Work out the finished part from the listing and answer in its coordinate system (mm). Face numbers are marked on the shaded views. A direction names the side the tool comes from. Coordinates: 2 decimals unless noted, no trailing zeros. Order: outer loops, then holes, each group sorted by start corner. A loop starts at its lowest first (then second) coordinate and runs counter-clockwise, first axis right, second up.
1. A tool of negligible diameter and unlimited length cuts with its end or side. For the marked faces 1 and 2, from which of +Z, -Z, +X, -X, +Y, -Y can it reach the whole face along a straight path? Write none if from no direction.
2. Find the intervals of material crossed by probe 1 along Y at (x, z) = (-5.5, 2); probe 2 along X at (y, z) = (0.5, 9); probe 3 along X at (y, z) = (4.25, 3.5), in increasing order.
3. The part is cut by section A-A, the plane y = 0. Give the vertices of the cut face in (x, z), then the cut area to 3 significant figures.
4. The part is cut by section B-B, the plane z = 3.5. Give the vertices of the cut face in (x, y), then the cut area to 3 significant figures.
5. Flat-ended cylindrical pins translate along their axes: pin 1 Ø4 at (y, z) = (-4, 5.5) entering from -X; pin 2 Ø1.5 at (x, y) = (-4.5, 1) entering from -Z; pin 3 Ø1.5 at (y, z) = (-4.5, 7) entering from -X. Find the tip coordinate at first contact, or state that the pin passes through.
```python
from build123d import *

# Parameters (mm, degrees)
SKETCH1_R           = 7.5
SKETCH1_R_2         = 5.05
BOSS_EXTRUDE1_DEPTH = 10
SKETCH2_W           = 6.1
SKETCH2_H           = 2.1
CUT_EXTRUDE1_DEPTH  = 16.229576488
CHAMFER1_SIZE       = 0.5
CHAMFER2_SIZE       = 0.5
CHAMFER3_SIZE       = 0.5


with BuildPart() as part:
    # Sketch1 → Boss-Extrude1 (new body)
    with BuildSketch(Plane.XY):
        with Locations((-1.2, 0)):
            Circle(SKETCH1_R)
        Circle(SKETCH1_R_2, mode=Mode.SUBTRACT)
    extrude(amount=BOSS_EXTRUDE1_DEPTH)

    # Sketch2 → Cut-Extrude1 (cut, through all)
    with BuildSketch(Plane.XY.offset(10)):
        with Locations((-3.05, 0)):
            Rectangle(SKETCH2_W, SKETCH2_H)
    extrude(amount=-CUT_EXTRUDE1_DEPTH, mode=Mode.SUBTRACT)

    # Chamfer1
    chamfer1_edges = [part.edges().sort_by_distance(p)[0] for p in [
        (5.05, 0, 10),
        (-5.519817807, -1.05, 10),
        (-5.519817807, 1.05, 10),
        (-6.1, 0, 10),
    ]]
    chamfer(chamfer1_edges, length=CHAMFER1_SIZE)

    # Chamfer2
    chamfer2_edges = [part.edges().sort_by_distance(p)[0] for p in [
        (5.05, 0, 0),
        (-5.519817807, -1.05, 0),
        (-6.1, 0, 0),
        (-5.519817807, 1.05, 0),
    ]]
    chamfer(chamfer2_edges, length=CHAMFER2_SIZE)

    # Chamfer3
    chamfer3_edges = [part.edges().sort_by_distance(p)[0] for p in [
        (-8.7, 0, 0),
        (-8.7, 0, 10),
    ]]
    chamfer(chamfer3_edges, length=CHAMFER3_SIZE)


solid = part.part
```
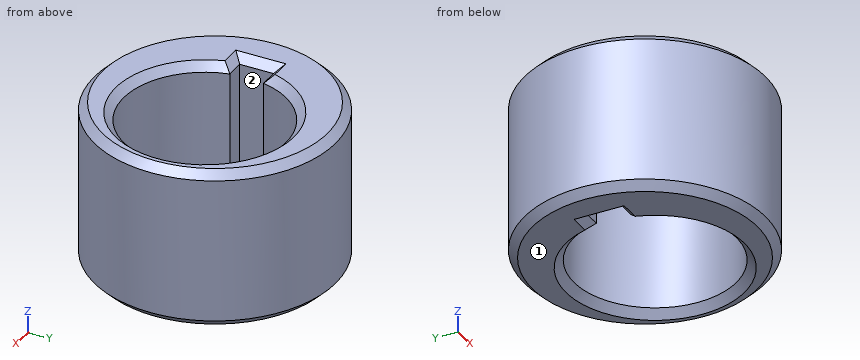
Geometry says:
1. face 1: -Z, +X, -X, +Y, -Y
1. face 2: +Z, -Z
2. probe 1: y = -6.14 to -1.05, 1.05 to 6.14
2. probe 2: x = -8.68 to -6.1, 5.03 to 6.28
2. probe 3: x = -7.38 to -2.73, 2.73 to 4.98
3. outline: (-8.7, 0.5) - (-8.2, 0) - (-6.6, 0) - (-6.1, 0.5) - (-6.1, 9.5) - (-6.6, 10) - (-8.2, 10) - (-8.7, 9.5) - close; (5.05, 0.5) - (5.55, 0) - (5.8, 0) - (6.3, 0.5) - (6.3, 9.5) - (5.8, 10) - (5.55, 10) - (5.05, 9.5) - close
3. area: 37.5 mm2
4. outline: circle Ø15 at (-1.2, 0); hole (-6.1, -1.05) - (-4.94, -1.05) arc R5.05 ccw (long way) to (-4.94, 1.05) - (-6.1, 1.05) - close
4. area: 94.3 mm2
5. pin 1: stops at x = -8.43
5. pin 2: stops at z = 0.21
5. pin 3: stops at x = -7.7
